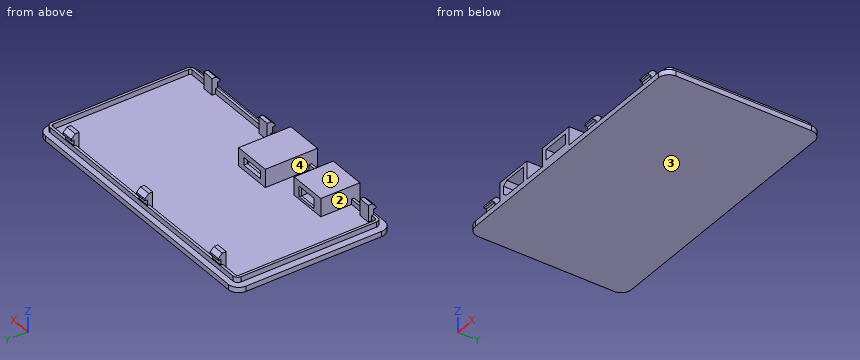
```python
from build123d import *

# Parameters (mm, degrees)
BOX096_W         = 10.8
BOX096_H         = 15
BOX096_DEPTH     = 5.6
CHAMFER007_SIZE2 = 1.8
CHAMFER007_SIZE  = 1.2
BOX097_W         = 8
BOX097_H         = 10
BOX097_DEPTH     = 4
BOX098_W         = 10.4
BOX098_H         = 18.5
BOX098_DEPTH     = 4
BOX099_W         = 9
BOX099_H         = 18
BOX099_DEPTH     = 3
BOX094_W         = 14.5
BOX094_H         = 15
BOX094_DEPTH     = 7
BOX095_W         = 14.5
BOX095_H         = 20
BOX095_DEPTH     = 7
BOX089_W         = 4.5
BOX089_H         = 2
BOX089_DEPTH     = 6
BOX090_W         = 4.5
BOX090_H         = 2
BOX090_DEPTH     = 6
BOX091_W         = 4.5
BOX091_H         = 2
BOX091_DEPTH     = 6
BOX086_W         = 4.5
BOX086_H         = 2
BOX086_DEPTH     = 6
BOX087_W         = 4.5
BOX087_H         = 2
BOX087_DEPTH     = 6
BOX088_W         = 4.5
BOX088_H         = 2
BOX088_DEPTH     = 6
BOX083_W         = 4.5
BOX083_H         = 3
BOX083_DEPTH     = 2.2
BOX084_W         = 4.5
BOX084_H         = 3
BOX084_DEPTH     = 2.2
BOX085_W         = 4.5
BOX085_H         = 3
BOX085_DEPTH     = 2.2
BOX080_W         = 4.5
BOX080_H         = 3
BOX080_DEPTH     = 2.2
BOX081_W         = 4.5
BOX081_H         = 3
BOX081_DEPTH     = 2.2
BOX082_W         = 4.5
BOX082_H         = 3
BOX082_DEPTH     = 2.2
CHAMFER006_SIZE  = 1.5
BOX079_W         = 107.6
BOX079_H         = 60
BOX079_DEPTH     = 2
FILLET015_R      = 4
BOX093_W         = 101.2
BOX093_H         = 53.6
BOX093_DEPTH     = 2
BOX092_W         = 103.2
BOX092_H         = 55.6
BOX092_DEPTH     = 2
FILLET016_1_R    = 1.8
FILLET016_2_R    = 0.8


with BuildPart() as chamfer007:
    # Box096 → Box096 (new body)
    with BuildSketch(Plane(origin=(19, 0, 0), x_dir=(1, 0, 0), z_dir=(0, 0, 1))):
        with Locations((5.4, 7.5)):
            Rectangle(BOX096_W, BOX096_H)
    extrude(amount=BOX096_DEPTH)

    # Chamfer007
    chamfer007_edges = [chamfer007.edges().sort_by_distance(p)[0] for p in [
        (19, 7.5, 5.6),
        (19, 7.5, 0),
    ]]
    chamfer007_side = chamfer007.faces().sort_by_distance((19, 7.5, 2.8))[0]
    chamfer(chamfer007_edges, length=CHAMFER007_SIZE, length2=CHAMFER007_SIZE2, reference=chamfer007_side)


with BuildPart() as chamfer007_1:
    # Chamfer007 placement: moved
    add(chamfer007.part.moved(Location((44.1, 33.4, -1.8))))


with BuildPart() as fusion058:
    # Box097 → Box097 (new body)
    with BuildSketch(Plane(origin=(65, 42, -1), x_dir=(1, 0, 0), z_dir=(0, 0, 1))):
        with Locations((4, 5)):
            Rectangle(BOX097_W, BOX097_H)
    extrude(amount=BOX097_DEPTH)

    # Fusion058: union Chamfer007
    add(chamfer007_1.part)


with BuildPart() as fusion058_1:
    # Fusion058 placement: moved
    add(fusion058.part.moved(Location((-0.05, 0, 0))))


with BuildPart() as cubo098:
    # Box098 → Box098 (new body)
    with BuildSketch(Plane.XY.offset(-0.1)):
        with Locations((5.2, 9.25)):
            Rectangle(BOX098_W, BOX098_H)
    extrude(amount=BOX098_DEPTH)


with BuildPart() as fusion061:
    # Box099 → Box099 (new body)
    with BuildSketch(Plane(origin=(0.7, 8, 0.4), x_dir=(1, 0, 0), z_dir=(0, 0, 1))):
        with Locations((4.5, 9)):
            Rectangle(BOX099_W, BOX099_H)
    extrude(amount=BOX099_DEPTH)

    # Fusion060: union Cubo098
    add(cubo098.part)


with BuildPart() as fusion061_1:
    # Fusion060 placement: moved
    add(fusion061.part.moved(Location((86.3, 34.3, -0.5))))

    # Fusion061: union Fusion058
    add(fusion058_1.part)


with BuildPart() as cubo094:
    # Box094 → Box094 (new body)
    with BuildSketch(Plane(origin=(61.2, 34.3, -2), x_dir=(1, 0, 0), z_dir=(0, 0, 1))):
        with Locations((7.25, 7.5)):
            Rectangle(BOX094_W, BOX094_H)
    extrude(amount=BOX094_DEPTH)


with BuildPart() as cubo095:
    # Box095 → Box095 (new body)
    with BuildSketch(Plane(origin=(84.3, 34.3, -2), x_dir=(1, 0, 0), z_dir=(0, 0, 1))):
        with Locations((7.25, 10)):
            Rectangle(BOX095_W, BOX095_H)
    extrude(amount=BOX095_DEPTH)


with BuildPart() as cubo089:
    # Box089 → Box089 (new body)
    with BuildSketch(Plane(origin=(0, -2, -5), x_dir=(1, 0, 0), z_dir=(0, 0, 1))):
        with Locations((2.25, 1)):
            Rectangle(BOX089_W, BOX089_H)
    extrude(amount=BOX089_DEPTH)


with BuildPart() as cubo090:
    # Box090 → Box090 (new body)
    with BuildSketch(Plane(origin=(40, -2, -5), x_dir=(1, 0, 0), z_dir=(0, 0, 1))):
        with Locations((2.25, 1)):
            Rectangle(BOX090_W, BOX090_H)
    extrude(amount=BOX090_DEPTH)


with BuildPart() as fusion054:
    # Box091 → Box091 (new body)
    with BuildSketch(Plane(origin=(80, -2, -5), x_dir=(1, 0, 0), z_dir=(0, 0, 1))):
        with Locations((2.25, 1)):
            Rectangle(BOX091_W, BOX091_H)
    extrude(amount=BOX091_DEPTH)

    # Fusion054: union Cubo089, Cubo090
    add(cubo089.part)
    add(cubo090.part)


with BuildPart() as fusion054_1:
    # Fusion054 placement: moved
    add(fusion054.part.moved(Location((55, 91.8, 2))))


with BuildPart() as cubo086:
    # Box086 → Box086 (new body)
    with BuildSketch(Plane(origin=(-5, 1, -5), x_dir=(1, 0, 0), z_dir=(0, 0, 1))):
        with Locations((2.25, 1)):
            Rectangle(BOX086_W, BOX086_H)
    extrude(amount=BOX086_DEPTH)


with BuildPart() as cubo087:
    # Box087 → Box087 (new body)
    with BuildSketch(Plane(origin=(50, 1, -5), x_dir=(1, 0, 0), z_dir=(0, 0, 1))):
        with Locations((2.25, 1)):
            Rectangle(BOX087_W, BOX087_H)
    extrude(amount=BOX087_DEPTH)


with BuildPart() as fusion055:
    # Box088 → Box088 (new body)
    with BuildSketch(Plane(origin=(80, 1, -5), x_dir=(1, 0, 0), z_dir=(0, 0, 1))):
        with Locations((2.25, 1)):
            Rectangle(BOX088_W, BOX088_H)
    extrude(amount=BOX088_DEPTH)

    # Fusion053: union Cubo086, Cubo087
    add(cubo086.part)
    add(cubo087.part)


with BuildPart() as fusion055_1:
    # Fusion053 placement: moved
    add(fusion055.part.moved(Location((55, 35.8, 2))))

    # Fusion055: union Fusion054
    add(fusion054_1.part)


with BuildPart() as cubo083:
    # Box083 → Box083 (new body)
    with BuildSketch(Plane(origin=(0, -2, 0.2), x_dir=(1, 0, 0), z_dir=(0, 0, 1))):
        with Locations((2.25, 1.5)):
            Rectangle(BOX083_W, BOX083_H)
    extrude(amount=BOX083_DEPTH)


with BuildPart() as cubo084:
    # Box084 → Box084 (new body)
    with BuildSketch(Plane(origin=(40, -2, 0.2), x_dir=(1, 0, 0), z_dir=(0, 0, 1))):
        with Locations((2.25, 1.5)):
            Rectangle(BOX084_W, BOX084_H)
    extrude(amount=BOX084_DEPTH)


with BuildPart() as fusion051:
    # Box085 → Box085 (new body)
    with BuildSketch(Plane(origin=(80, -2, 0.2), x_dir=(1, 0, 0), z_dir=(0, 0, 1))):
        with Locations((2.25, 1.5)):
            Rectangle(BOX085_W, BOX085_H)
    extrude(amount=BOX085_DEPTH)

    # Fusion051: union Cubo083, Cubo084
    add(cubo083.part)
    add(cubo084.part)


with BuildPart() as fusion051_1:
    # Fusion051 placement: moved
    add(fusion051.part.moved(Location((55, 91.8, 2))))


with BuildPart() as cubo080:
    # Box080 → Box080 (new body)
    with BuildSketch(Plane(origin=(-5, 0, 0.2), x_dir=(1, 0, 0), z_dir=(0, 0, 1))):
        with Locations((2.25, 1.5)):
            Rectangle(BOX080_W, BOX080_H)
    extrude(amount=BOX080_DEPTH)


with BuildPart() as cubo081:
    # Box081 → Box081 (new body)
    with BuildSketch(Plane(origin=(50, 0, 0.2), x_dir=(1, 0, 0), z_dir=(0, 0, 1))):
        with Locations((2.25, 1.5)):
            Rectangle(BOX081_W, BOX081_H)
    extrude(amount=BOX081_DEPTH)


with BuildPart() as chamfer006:
    # Box082 → Box082 (new body)
    with BuildSketch(Plane(origin=(80, 0, 0.2), x_dir=(1, 0, 0), z_dir=(0, 0, 1))):
        with Locations((2.25, 1.5)):
            Rectangle(BOX082_W, BOX082_H)
    extrude(amount=BOX082_DEPTH)

    # Fusion050: union Cubo080, Cubo081
    add(cubo080.part)
    add(cubo081.part)


with BuildPart() as chamfer006_1:
    # Fusion050 placement: moved
    add(chamfer006.part.moved(Location((55, 35.8, 2))))

    # Fusion052: union Fusion051
    add(fusion051_1.part)

    # Fusion056: union Fusion055
    add(fusion055_1.part)

    # Chamfer006
    chamfer006_edges = [chamfer006_1.edges().sort_by_distance(p)[0] for p in [
        (137.25, 35.8, 4.4),
        (52.25, 35.8, 4.4),
        (107.25, 35.8, 4.4),
        (137.25, 92.8, 4.4),
        (57.25, 92.8, 4.4),
        (97.25, 92.8, 4.4),
    ]]
    chamfer(chamfer006_edges, length=CHAMFER006_SIZE)


with BuildPart() as chamfer006_2:
    # Chamfer006 placement: moved
    add(chamfer006_1.part.moved(Location((0.25, 0, 0))))


with BuildPart() as fillet015:
    # Box079 → Box079 (new body)
    with BuildSketch(Plane(origin=(43.7, 34.3, -4), x_dir=(1, 0, 0), z_dir=(0, 0, 1))):
        with Locations((53.8, 30)):
            Rectangle(BOX079_W, BOX079_H)
    extrude(amount=BOX079_DEPTH)

    # Fillet015
    fillet015_edges = [fillet015.edges().sort_by_distance(p)[0] for p in [
        (43.7, 34.3, -3),
        (43.7, 94.3, -3),
        (151.3, 34.3, -3),
        (151.3, 94.3, -3),
    ]]
    fillet(fillet015_edges, radius=FILLET015_R)


with BuildPart() as cubo093:
    # Box093 → Box093 (new body)
    with BuildSketch(Plane(origin=(49.7, 35.3, -2), x_dir=(1, 0, 0), z_dir=(0, 0, 1))):
        with Locations((50.6, 26.8)):
            Rectangle(BOX093_W, BOX093_H)
    extrude(amount=BOX093_DEPTH)


with BuildPart() as base:
    # Box092 → Box092 (new body)
    with BuildSketch(Plane(origin=(48.7, 34.3, -2), x_dir=(1, 0, 0), z_dir=(0, 0, 1))):
        with Locations((51.6, 27.8)):
            Rectangle(BOX092_W, BOX092_H)
    extrude(amount=BOX092_DEPTH)

    # Cut019: cut Cubo093
    add(cubo093.part, mode=Mode.SUBTRACT)

    # Fillet016 1
    fillet016_1_edges = [base.edges().sort_by_distance(p)[0] for p in [
        (48.7, 34.3, -1),
        (48.7, 89.9, -1),
        (151.9, 34.3, -1),
        (151.9, 89.9, -1),
    ]]
    fillet(fillet016_1_edges, radius=FILLET016_1_R)

    # Fillet016 2
    fillet016_2_edges = [base.edges().sort_by_distance(p)[0] for p in [
        (150.9, 35.3, -1),
        (49.7, 35.3, -1),
        (150.9, 88.9, -1),
        (49.7, 88.9, -1),
    ]]
    fillet(fillet016_2_edges, radius=FILLET016_2_R)


with BuildPart() as base_1:
    # Fillet016 placement: moved
    add(base.part.moved(Location((-2.2, 2.2, 0))))

    # Fusion057: union Chamfer006, Fillet015
    add(chamfer006_2.part)
    add(fillet015.part)

    # Fusion059: union Cubo094, Cubo095
    add(cubo094.part)
    add(cubo095.part)

    # Cut020: cut Fusion061
    add(fusion061_1.part, mode=Mode.SUBTRACT)


with BuildPart() as base_2:
    # Cut020 placement: moved
    add(base_1.part.moved(Location((0, 0, -5))))


solid = base_2.part
```
Design review of the part built by this model. Coordinates are the model's own, in mm. Face numbers are marked on the shaded views. A direction names the side the tool comes from. Round coordinates to 2 decimals unless told otherwise and drop trailing zeros. Order: outer loops, then holes, each group sorted by start corner. A loop starts at its lowest first (then second) coordinate and runs counter-clockwise, first axis right, second up. Notation, with made-up numbers: (81.5, -5.75) - (115.5, -5.75) arc R24 cw to (115.5, 21.25) - close; hole circle Ø5 at (56.25, 13.25). An arc over 180 degrees is marked (long way). Return JSON: item names as keys, results as strings.
Q1. Consider section A-A on y = 44. Give the number of separate pieces and of enclosed holes in the cut face, plus the area to 3 significant figures.
Computed values:
{"separate pieces": "1", "enclosed holes": "2", "area": "322 mm2"}
Q2. Consider section B-B on x = 103. Write out the cut boundary in (y, z), plus the area to 3 significant figures.
Computed values:
{"outline": "(34.3, -9) - (94.3, -9) - (94.3, -7) - (92.1, -7) - (92.1, -5) - (91.1, -5) - (91.1, -7) - (37.5, -7) - (37.5, -5) - (36.5, -5) - (36.5, -7) - (34.3, -7) - close", "area": "124 mm2"}
Q3. The part is to be moulded in two halves that separate along X. For the marked faces 3 and 4, say which applies: pulls with the +X half, pulls with the -X half, needs draft (parallel to the pull), parting line crosses it, or undercut.
Computed values:
{"face 3": "needs draft", "face 4": "undercut"}
Q4. Consider section C-C on y = 59. Write out the cut boundary in (x, z), plus the area to 3 significant figures.
Computed values:
{"outline": "(43.7, -9) - (151.3, -9) - (151.3, -7) - (149.7, -7) - (149.7, -5) - (148.7, -5) - (148.7, -7) - (47.5, -7) - (47.5, -5) - (46.5, -5) - (46.5, -7) - (43.7, -7) - close", "area": "219 mm2"}
Q5. For pin 1 Ø4 at (x, z) = (135.5, -6) entering from -Y; pin 2 Ø1.6 at (y, z) = (43, -4.5) entering from +X; pin 3 Ø1.6 at (x, y) = (52.5, 38) entering from +Z; pin 4 Ø1.5 at (y, z) = (37, -2.5) entering from -X, all flat-tipped, find the tip position at first contact; note any pin that passes through.
Computed values:
{"pin 1": "stops at y = 34.3", "pin 2": "stops at x = 149.7", "pin 3": "stops at z = -0.6", "pin 4": "stops at x = 50.25"}
Q6. Machinability: for the marked faces 1 and 2, which of the approach directions +Z, -Z, +X, -X, +Y, -Y give a long, thin tool a straight path to every point of the face, cutting with its end or side? Answer none if there is none.
Computed values:
{"face 1": "+Z, +X, -X, +Y, -Y", "face 2": "+Z"}
Q7. Wall thickness on L1, parallel to X at y = 51, z = -6.25; L2, parallel to X at y = 44, z = -4; L3, parallel to Y at x = 89.5, z = -5.5: over which ranges is each line inside the solid? List them lowest first. Write a range as [from, to].
Computed values:
{"L1": "x = [46.5, 47.5], [84.3, 98.8], [148.7, 149.7]", "L2": "x = [61.2, 63.05], [73.85, 75.7], [84.3, 86.3], [96.7, 98.8]", "L3": "y = [52.8, 54.3], [91.1, 92.1]"}
